from build123d import *

# Parameters (mm, degrees)
F0_W         = 914.4
F0_H         = 2438.4
F1_DEPTH     = 609.6
F3_T         = -2.54
F4_T1_DEPTH  = 2433.32
F4_T3_DEPTH  = 909.32
F4_T9_DEPTH  = 2446.02
F4_T15_DEPTH = 922.02
F4_T24_DEPTH = 2446.02
F4_T30_DEPTH = 922.02


# Not quite as in the source:
# - a fillet or chamfer that OpenCascade refuses, or shapes differently, is made with other operations: its cross-section is extruded or revolved along the edge and cut away or added


with BuildPart() as f1:
    # F0 (on Top) → F1 (new body)
    with BuildSketch(Plane.XY):
        with Locations((-243.063261795, 394.9879257202)):
            Rectangle(F0_W, F0_H)
    extrude(amount=F1_DEPTH)

    # F3
    f3_openings = [f1.faces().sort_by_distance(p)[0] for p in [
        (-243.063262, 394.987926, 609.6),
    ]]
    offset(amount=F3_T, openings=f3_openings)

    # F4: fillet of radius 5.08 on 3 edges, made by hand

    # F4_s2 → F4_t1 (cut)
    with BuildSketch(Plane.XZ.offset(-1611.6479257202)):
        with BuildLine():
            ThreePointArc((-702.803261795, 609.6), (-699.2111593466, 608.1121024484), (-697.723261795, 604.52))
            Line((-697.723261795, 604.52), (-697.723261795, 609.6))
            Line((-697.723261795, 609.6), (-702.803261795, 609.6))
        make_face()
    extrude(amount=F4_T1_DEPTH, mode=Mode.SUBTRACT)

    # F4_s4 → F4_t3 (cut)
    with BuildSketch(Plane.YZ.offset(-697.723261795)):
        with BuildLine():
            ThreePointArc((-826.7520742798, 609.6), (-823.1599718314, 608.1121024484), (-821.6720742798, 604.52))
            Line((-821.6720742798, 604.52), (-821.6720742798, 609.6))
            Line((-821.6720742798, 609.6), (-826.7520742798, 609.6))
        make_face()
        with BuildLine():
            ThreePointArc((1616.7279257202, 609.6), (1613.1358232718, 608.1121024484), (1611.6479257202, 604.52))
            Line((1611.6479257202, 604.52), (1611.6479257202, 609.6))
            Line((1611.6479257202, 609.6), (1616.7279257202, 609.6))
        make_face()
    extrude(amount=F4_T3_DEPTH, mode=Mode.SUBTRACT)


with BuildPart() as f4_tool7:
    # F4_s8 → F4_t9 (new body)
    with BuildSketch(Plane.XZ.offset(-1624.3479257202)):
        with BuildLine():
            ThreePointArc((-702.803261795, 609.6), (-699.2111593466, 608.1121024484), (-697.723261795, 604.52))
            Line((-697.723261795, 604.52), (-697.723261795, 609.6))
            Line((-697.723261795, 609.6), (-702.803261795, 609.6))
        make_face()
    extrude(amount=F4_T9_DEPTH)

    split(bisect_by=Plane.YZ.offset(-700.263261795), keep=Keep.TOP)

    split(bisect_by=Plane.XZ.offset(-1614.1879257202), keep=Keep.TOP)

    split(bisect_by=Plane.XZ.offset(-1611.6479257202), keep=Keep.BOTTOM)


with BuildPart() as f4_tool13:
    # F4_s14 → F4_t15 (new body)
    with BuildSketch(Plane.YZ.offset(211.596738205)):
        with BuildLine():
            ThreePointArc((1616.7279257202, 609.6), (1613.1358232718, 608.1121024484), (1611.6479257202, 604.52))
            Line((1611.6479257202, 604.52), (1611.6479257202, 609.6))
            Line((1611.6479257202, 609.6), (1616.7279257202, 609.6))
        make_face()
    extrude(amount=-F4_T15_DEPTH)

    split(bisect_by=Plane.YZ.offset(-700.263261795), keep=Keep.TOP)

    split(bisect_by=Plane.XZ.offset(-1614.1879257202), keep=Keep.TOP)

    split(bisect_by=Plane.YZ.offset(-697.723261795), keep=Keep.BOTTOM)


with BuildPart() as f4_tool7_1:
    add(f4_tool7.part)

    # F4_t19: intersect F4_tool13
    add(f4_tool13.part, mode=Mode.INTERSECT)


with BuildPart() as f1_1:
    add(f1.part)

    # F4_t5: cut F4_tool7
    add(f4_tool7_1.part, mode=Mode.SUBTRACT)


with BuildPart() as f4_tool22:
    # F4_s23 → F4_t24 (new body)
    with BuildSketch(Plane.XZ.offset(-1611.6479257202)):
        with BuildLine():
            ThreePointArc((-702.803261795, 609.6), (-699.2111593466, 608.1121024484), (-697.723261795, 604.52))
            Line((-697.723261795, 604.52), (-697.723261795, 609.6))
            Line((-697.723261795, 609.6), (-702.803261795, 609.6))
        make_face()
    extrude(amount=F4_T24_DEPTH)

    split(bisect_by=Plane.YZ.offset(-700.263261795), keep=Keep.TOP)

    split(bisect_by=Plane.XZ.offset(824.2120742798), keep=Keep.BOTTOM)

    split(bisect_by=Plane.XZ.offset(821.6720742798), keep=Keep.TOP)


with BuildPart() as f4_tool28:
    # F4_s29 → F4_t30 (new body)
    with BuildSketch(Plane.YZ.offset(-710.423261795)):
        with BuildLine():
            ThreePointArc((-826.7520742798, 609.6), (-823.1599718314, 608.1121024484), (-821.6720742798, 604.52))
            Line((-821.6720742798, 604.52), (-821.6720742798, 609.6))
            Line((-821.6720742798, 609.6), (-826.7520742798, 609.6))
        make_face()
    extrude(amount=F4_T30_DEPTH)

    split(bisect_by=Plane.YZ.offset(-700.263261795), keep=Keep.TOP)

    split(bisect_by=Plane.XZ.offset(824.2120742798), keep=Keep.BOTTOM)

    split(bisect_by=Plane.YZ.offset(-697.723261795), keep=Keep.BOTTOM)


with BuildPart() as f4_tool22_1:
    add(f4_tool22.part)

    # F4_t34: intersect F4_tool28
    add(f4_tool28.part, mode=Mode.INTERSECT)


with BuildPart() as f1_2:
    add(f1_1.part)

    # F4_t20: cut F4_tool22
    add(f4_tool22_1.part, mode=Mode.SUBTRACT)


solid = f1_2.part
Geometry: final body of the model. Coordinates: model frame, mm. A direction names the side the tool comes from. Round coordinates to 2 decimals unless told otherwise and drop trailing zeros. Loops run counter-clockwise (first coordinate to the right, second up) from the corner with the lowest first, then second, coordinate; pieces in that order, holes last. Notation, with made-up numbers: (25.25, 0.25) - (44.25, 0.25) arc R21 ccw to (44.25, 38.25) - close; hole circle Ø6 at (66, 23.5). An arc over 180 degrees is marked (long way). Write each question's results on one line, items separated by ' | '. Start each with the question number.
1) Cut plane C-C on y = -415. Return loops of the section in (x, z).
2) Cut plane B-B on x = -616. Return loops of the section in (y, z).
3) Mould query, pull axis X, two halves, no side actions, for faces 3 (the face through (214.137, 378, 301)), 4 (the face through (-249, 1614.188, 301)), 5 (the face through (-249, -821.672, 308)). Classes: released by +X, released by -X, zero draft, split by the parting line, or undercut.
4) Line query: probe 1 along Y at (x, z) = (41, 108); probe 2 along X at (y, z) = (628.5, 342); probe 3 along Z at (x, y) = (-92, 863.5). Output: solid intervals per line, ascending. Write a range as [from, to].
5) Access query for faces 1 (the face through (-700.263, 378, 300)), 2 (the face through (-249, 1611.648, 308)). Directions: +Z, -Z, +X, -X, +Y, -Y. A direction counts if a zero-diameter tool reaches every point of the face in a straight line with its end or side. Return the directions, or none.
6) First-contact query: P1, Ø8, axis at x = -470.5, y = 270.5, coming from the +Z side. Flat tip, straight axial feed; report the tip coordinate or a pass-through.
7) Cut plane A-A on z = 347. Return loops of the section in (x, y), then the cut area to 3 significant figures.
Verdict:
1) outline: (-700.26, 0) - (214.14, 0) - (214.14, 609.6) - (211.6, 609.6) - (211.6, 2.54) - (-697.72, 2.54) - (-697.72, 604.52) arc R5.08 ccw to (-700.26, 608.92) - close
2) outline: (-824.21, 0) - (1614.19, 0) - (1614.19, 608.92) arc R5.08 ccw to (1611.65, 604.52) - (1611.65, 2.54) - (-821.67, 2.54) - (-821.67, 604.52) arc R5.08 ccw to (-824.21, 608.92) - close
3) face 3: released by +X | face 4: zero draft | face 5: undercut
4) probe 1: y = [-824.21, -821.67], [1611.65, 1614.19] | probe 2: x = [-700.26, -697.72], [211.6, 214.14] | probe 3: z = [0, 2.54]
5) face 1: +Z, -Z, -X, +Y, -Y | face 2: +Z
6) P1: stops at z = 2.54
7) outline: (-700.26, -824.21) - (214.14, -824.21) - (214.14, 1614.19) - (-700.26, 1614.19) - close; hole (-697.72, -821.67) - (211.6, -821.67) - (211.6, 1611.65) - (-697.72, 1611.65) - close | area: 17,000 mm2
